For this review, take the finished solid that the model builds, in its own axes (mm). A direction names the side the tool comes from. Round coordinates to 2 decimals unless told otherwise and drop trailing zeros. Order: outer loops, then holes, each group sorted by start corner. A loop starts at its lowest first (then second) coordinate and runs counter-clockwise, first axis right, second up. Notation, with made-up numbers: M 81,6.25 L 129,6.25 A34 ccw 129,36.25 Z; hole C 72,-1.75 d5. An arc over 180 degrees is marked long. Answer in a Markdown table with one row per item. Add a question column.
```python
from build123d import *

# Parameters (mm, degrees)
F0_W     = 20
F0_H     = 60
F1_DEPTH = 7.5
F2_W     = 5.122859
F2_H     = 5.811491
F2_W_2   = 4.621518
F2_W_3   = 5
F2_H_2   = 5
F3_DEPTH = 15


with BuildPart() as f1:
    # F0 (on Top) → F1 (new body)
    with BuildSketch(Plane.XY):
        with Locations((4.877141, 11.942423)):
            Rectangle(F0_W, F0_H)
    extrude(amount=F1_DEPTH)

    # F2 (on face) → F3 (join)
    with BuildSketch(Plane(origin=(0, 0, 0), x_dir=(1, 0, 0), z_dir=(0, 0, -1))):
        with Locations((-2.56143, 15.151832)):
            Rectangle(F2_W, F2_H)
        with Locations((12.566382, 15.151832)):
            Rectangle(F2_W_2, F2_H)
        with Locations((12.377141, -39.442423)):
            Rectangle(F2_W_3, F2_H_2)
        with Locations((-2.56143, -39.442423)):
            Rectangle(F2_W, F2_H_2)
    extrude(amount=F3_DEPTH)


solid = f1.part
```
1. Consider section B-B on x = 6. Write out the cut boundary in (y, z), plus the area to 3 significant figures.
2. Consider section C-C on y = 22.5. Write out the cut boundary in (x, z).
3. Clearance check with a flat-ended pin moving along its axis: pin 1 Ø1 at (x, y) = (-1, 19.5) entering from -Z. State where the tip first meets the part, or that it passes through.
4. For faces 4 (the flat face through (10.256, -15, -7)), 5 (the flat face through (12, 36.942, -7)), 6 (the flat face through (0, -15, -7)), list the 3-axis set-ups (+Z, -Z, +X, -X, +Y, -Y) from which the entire face can be reached by the end or side of a thin tool; tool diameter is ignored.
5. To check wall thickness, follow probe 1 along X at (y, z) = (39.5, -2); probe 2 along X at (y, z) = (-15, -10.75); probe 3 along Y at (x, z) = (-0.5, -5.75). State the ranges of each line that lie inside material, in increasing order. Write a range as [from, to].
6. Consider section A-A on z = -2.25. Write out the cut boundary in (x, y), plus the area to 3 significant figures.
7. The part is to be moulded in two halves that separate along Y. For faces 1 (the flat face through (5, -18.058, 4)), 2 (the flat face through (13, -12.246, -7)), 3 (the flat face through (0, 39, -7)), say which applies: pulls with the +Y half, pulls with the -Y half, needs draft (parallel to the pull), parting line crosses it, or undercut.
Solved:
| question | item | result |
|---|---|---|
| 1 | outline | M -18.06,0 L 41.94,0 L 41.94,7.5 L -18.06,7.5 Z |
| 1 | area | 450 mm^2 |
| 2 | outline | M -5.12,0 L 14.88,0 L 14.88,7.5 L -5.12,7.5 Z |
| 3 | pin 1 | stops at z = 0 |
| 4 | face 4 | -Z, -Y |
| 4 | face 5 | -Z, +X, -X |
| 4 | face 6 | -Z, +Y, -Y |
| 5 | probe 1 | x = [-5.12, 0], [9.88, 14.88] |
| 5 | probe 2 | x = [-5.12, 0], [10.26, 14.88] |
| 5 | probe 3 | y = [-18.06, -12.25], [36.94, 41.94] |
| 6 | outline | M -5.12,-18.06 L 0,-18.06 L 0,-12.25 L -5.12,-12.25 Z; M -5.12,36.94 L 0,36.94 L 0,41.94 L -5.12,41.94 Z; M 9.88,36.94 L 14.88,36.94 L 14.88,41.94 L 9.88,41.94 Z; M 10.26,-18.06 L 14.88,-18.06 L 14.88,-12.25 L 10.26,-12.25 Z |
| 6 | area | 107 mm^2 |
| 7 | face 1 | pulls with the -Y half |
| 7 | face 2 | undercut |
| 7 | face 3 | needs draft |
